Geometry: final body of the model. Coordinates: model frame, mm. A direction names the side the tool comes from. Give positions to 0.01 mm unless a question says otherwise; leave off trailing zeros. Write each loop counter-clockwise with the first axis right and the second up, starting at its lowest first coordinate (ties: lowest second). Pieces come first, ordered by that corner, then holes.
Q1. Line query: L1, parallel to Y at x = -4.25, z = -35.5; L2, parallel to X at y = 19.5, z = -20; L3, parallel to Y at x = -6.5, z = -28.5. Output: solid intervals per line, ascending.
Q2. Reachability of faces 1 (the face through (0, 32, -39)), 2 (the face through (4, 16, -31)), 3 (the face through (-8, 23, -34)) from +Z, -Z, +X, -X, +Y, -Y: full face, straight path, thin tool, end or side. Return the list, or none.
Q3. Cut plane D-D on z = -28.5. Return the cut outline in (x, y).
Q4. Draft query along Y for faces 4 (the face through (0, 0, -22)), 5 (the face through (-13, 5, -22)), 6 (the face through (-4, 16, -31)), 7 (the face through (9, 23, -34)). Return one class per face: pulls with the +Y half, pulls with the -Y half, needs draft (parallel to the pull), parting line crosses it, or undercut.
Q5. Cut plane C-C on y = 11. Return the cut outline in (x, z), plus the area to 3 significant figures.
Q6. Pin query (flat end, axial travel): pin 1 (3 mm diameter, centred on x = -2, z = -20, fed in from +Y); pin 2 (4.5 mm diameter, centred on x = 9.5, z = -24, fed in from +Y); pin 3 (7 mm diameter, centred on y = 14.5, z = -27, fed in from -X). Return the tip coordinate at first contact, or that it passes through.
Q7. Cut plane A-A on z = -20. Return the cut outline in (x, y), plus the area to 3 significant figures.
Q8. Cut plane B-B on x = -7.5. Return the cut outline in (y, z), plus the area to 3 significant figures.
```python
from build123d import *

# Parameters (mm, degrees)
EXTRUDE_1_DEPTH     = 13
SKETCH_2_W          = 9
SKETCH_2_H          = 14
CUT_EXTRUDE_1_DEPTH = 57.727418415


with BuildPart() as part:
    # 草图1 → 凸台-拉伸1 (new, symmetric)
    with BuildSketch(Plane(origin=(0, 0, 0), x_dir=(0, 0, -1), z_dir=(1, 0, 0))):
        Polygon((0, 0), (45, 0), (45, 32), (32, 32), align=None)
    extrude(amount=EXTRUDE_1_DEPTH, both=True)

    # 草图2 → 切除-拉伸1 (cut, through all)
    with BuildSketch(Plane(origin=(0, 0, -45), x_dir=(-1, 0, 0), z_dir=(0, 0, -1))):
        with Locations((-8.5, 16)):
            Rectangle(SKETCH_2_W, SKETCH_2_H)
        with Locations((8.5, 16)):
            Rectangle(SKETCH_2_W, SKETCH_2_H)
    extrude(amount=-CUT_EXTRUDE_1_DEPTH, mode=Mode.SUBTRACT)


solid = part.part
```
Data:
1. L1: y = 0 to 9, 23 to 32
1. L2: x = -4 to 4
1. L3: y = 0 to 9, 23 to 28.5
2. face 1: +Z, -Z, +X, -X, +Y
2. face 2: +Z, -Z, +X
2. face 3: +Z, -Z, -X
3. outline: (-13, 0) - (13, 0) - (13, 9) - (4, 9) - (4, 23) - (13, 23) - (13, 28.5) - (-13, 28.5) - (-13, 23) - (-4, 23) - (-4, 9) - (-13, 9) - close
4. face 4: pulls with the -Y half
4. face 5: needs draft
4. face 6: undercut
4. face 7: undercut
5. outline: (-4, -45) - (4, -45) - (4, -11) - (-4, -11) - close
5. area: 272 mm2
6. pin 1: stops at y = 21.5
6. pin 2: stops at y = 26.25
6. pin 3: stops at x = -4
7. outline: (-13, 0) - (13, 0) - (13, 9) - (4, 9) - (4, 20) - (-4, 20) - (-4, 9) - (-13, 9) - close
7. area: 322 mm2
8. outline: (0, -45) - (9, -45) - (9, -9) - (0, 0) - close; (23, -45) - (32, -45) - (32, -32) - (23, -23) - close
8. area: 522 mm2
